Work out the finished part from the listing and answer in its coordinate system (mm). A direction names the side the tool comes from. Coordinates: 2 decimals unless noted, no trailing zeros. Loops run counter-clockwise (first coordinate to the right, second up) from the corner with the lowest first, then second, coordinate; pieces in that order, holes last. Notation, with made-up numbers: M 45,-7.75 L 103,-7.75 A17 cw 103,22.25 Z; hole C -35.5,56 d3. An arc over 180 degrees is marked long. Write each question's results on one line, items separated by ' | '.
```python
from build123d import *

# Parameters (mm, degrees)
SKETCH_1_W          = 100
SKETCH_1_H          = 100
EXTRUDE_1_DEPTH     = 8
SKETCH_2_OUTSIDE_W  = 130.33
SKETCH_2_OUTSIDE_H  = 130.33
CUT_EXTRUDE_1_DEPTH = 142.647449677
SKETCH_3_R          = 1.5
CUT_EXTRUDE_2_DEPTH = 133.94238179


with BuildPart() as part:
    # 草图1 → 凸台-拉伸1 (new body)
    with BuildSketch(Plane.XY):
        with Locations((50, 50)):
            Rectangle(SKETCH_1_W, SKETCH_1_H)
    extrude(amount=EXTRUDE_1_DEPTH)

    # 草图2 outside → 切除-拉伸1 (cut, through all)
    with BuildSketch(Plane.XY.offset(8)):
        with Locations((50, 50)):
            Rectangle(SKETCH_2_OUTSIDE_W, SKETCH_2_OUTSIDE_H)
        with BuildLine():
            Line((90, 97.517572139), (90, 55.3))
            ThreePointArc((90, 55.3), (48.097501561, 19.250031211), (10, 59.3))
            Line((10, 59.3), (10, 97.517572139))
            Line((10, 97.517572139), (90, 97.517572139))
        make_face(mode=Mode.SUBTRACT)
    extrude(amount=-CUT_EXTRUDE_1_DEPTH, mode=Mode.SUBTRACT)

    # 草图3 → 切除-拉伸2 (cut, through all)
    with BuildSketch(Plane.XY.offset(8)):
        with Locations((75, 84.3)):
            Circle(SKETCH_3_R)
        with Locations(Location((75, 34.3, 0), (0, 0, 180))):
            Circle(SKETCH_3_R)
        with Locations((25, 34.3)):
            Circle(SKETCH_3_R)
        with Locations(Location((25, 84.3, 0), (0, 0, 180))):
            Circle(SKETCH_3_R)
        with BuildLine():
            Line((29.478409373, 68.3), (22.1, 68.3))
            Line((22.1, 68.3), (22.1, 50.3))
            Line((22.1, 50.3), (29.478409373, 50.3))
            ThreePointArc((29.478409373, 50.3), (72.6, 59.3), (29.478409373, 68.3))
        make_face()
    extrude(amount=-CUT_EXTRUDE_2_DEPTH, mode=Mode.SUBTRACT)


solid = part.part
```
1) Find section D-D, the plane y = 45. Give the vertices of the cut face in (x, z), and give its area (3 significant figures).
Check result:
outline: M 12.64,0 L 32.73,0 L 32.73,8 L 12.64,8 Z; M 67.47,0 L 87.56,0 L 87.56,8 L 67.47,8 Z | area: 321 mm^2
2) Find section C-C, the plane y = 84.3. Give the vertices of the cut face in (x, z), and give its area (3 significant figures).
Check result:
outline: M 10,0 L 23.5,0 L 23.5,8 L 10,8 Z; M 26.5,0 L 73.5,0 L 73.5,8 L 26.5,8 Z; M 76.5,0 L 90,0 L 90,8 L 76.5,8 Z | area: 592 mm^2
3) Find section B-B, the plane x = 50.1. Give the vertices of the cut face in (y, z).
Check result:
outline: M 19.2,0 L 36.8,0 L 36.8,8 L 19.2,8 Z; M 81.8,0 L 97.52,0 L 97.52,8 L 81.8,8 Z
4) For a pull along Y with two mould halves and no side action, classify faces 3 (the face through (26, 68.3, 4)), 4 (the face through (48.951, 19.216, 4.056)), 5 (the face through (10, 78, 4)) as released by +Y, released by -Y, zero draft, split by the parting line, or undercut.
Check result:
face 3: undercut | face 4: released by -Y | face 5: zero draft
5) Which of the six approach directions +Z, -Z, +X, -X, +Y, -Y give full straight-line access (tool end or side, diameter ignored) to faces 1 (the face through (67, 76, 8)), 2 (the face through (22.1, 59, 4))?
Check result:
face 1: +Z, +X, -X, +Y, -Y | face 2: +Z, -Z
6) Straight lines are drawn through the part: probe 1 along X at (y, z) = (84.3, 3); probe 2 along Y at (x, z) = (50.1, 3); probe 3 along X at (y, z) = (34.5, 0.5). For each, find the intervals that lie inside material, in ascending order. Write a range as [from, to].
Check result:
probe 1: [10, 23.5], [26.5, 73.5], [76.5, 90] | probe 2: [19.2, 36.8], [81.8, 97.52] | probe 3: [18.59, 23.51], [26.49, 73.51], [76.49, 81.61]
7) Given pin 1 Ø2 at (y, z) = (53, 6) entering from +X; pin 2 Ø1 at (y, z) = (58, 6.5) entering from -X; pin 3 Ø5 at (x, y) = (25, 84.3) entering from -Z; pin 4 Ø3.5 at (x, z) = (27, 3.5) entering from -Y, each flat-ended and moving along its own axis, determine where each tip first touches the part or whether it passes through.
Check result:
pin 1: x = 89.85 | pin 2: x = 10.01 | pin 3: z = 0 | pin 4: y = 25.36
8) Find section A-A, the plane z = 3.25. Give the vertices of the cut face in (x, y).
Check result:
outline: M 10,59.3 A40.1 ccw 90,55.3 L 90,97.52 L 10,97.52 Z; hole M 22.1,50.3 L 29.48,50.3 A22.5 ccw long 29.48,68.3 L 22.1,68.3 Z; hole C 25,34.3 d3; hole C 25,84.3 d3; hole C 75,34.3 d3; hole C 75,84.3 d3
